For this review, take the finished solid that the model builds, in its own axes (mm). Give positions to 0.01 mm unless a question says otherwise; leave off trailing zeros. Loops run counter-clockwise (first coordinate to the right, second up) from the corner with the lowest first, then second, coordinate; pieces in that order, holes last. Notation, with made-up numbers: (78.25, -7.75) - (124.25, -7.75) arc R11 ccw to (124.25, 5.25) - close; hole circle Ø2 at (88, 51.5). An arc over 180 degrees is marked (long way). Answer in a Markdown table with one row per item.
Autodesk Inventor part; units mm, degrees
ref_plane "YZ Plane" through (0, 0, 0) normal (1, 0, 0) x (0, 1, 0)
ref_plane "XZ Plane" through (0, 0, 0) normal (0, 1, 0) x (-1, 0, 0)
ref_plane "XY Plane" through (0, 0, 0) normal (0, 0, 1) x (1, 0, 0)
sketch "Sketch1" plane through (0, 0, 0) normal (0, 0, 1) x (1, 0, 0)
  line L0 (0, 0) -> (0, 79.375)
  line L1 (0, 79.375) -> (-50.8, 79.375)
  line L2 (-50.8, 79.375) -> (-50.8, 25.4)
  line L3 (-50.8, 25.4) -> (-50.8, 0)
  line L4 (-50.8, 0) -> (0, 0)
  circle A0 centre (-25.4, 53.975) radius 6.35
  dimension "d0" = 79.375
  dimension "d1" = 50.8
  dimension "d2" = 25.4
  dimension "d3" = 50.8
  dimension "d4" = 25.4
  dimension "d5" = 25.4
  dimension "d6" = 12.7
extrude "Extrusion1" add sketch "Sketch1" against normal blind 3.175
properties part number "gearmotor mounting plate"
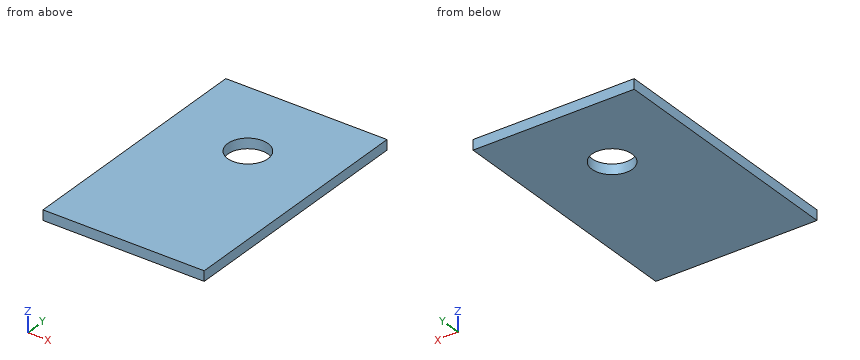
1. We need section C-C, the plane z = -2.6. Give the boundary of the cut face in (x, y) (3 decimals).
Values:
| item | result |
|---|---|
| outline | (-50.8, 0) - (0, 0) - (0, 79.375) - (-50.8, 79.375) - close; hole circle Ø12.7 at (-25.4, 53.975) |
2. Wall thickness on line 1 (Y direction, x = -25.4, z = -1.15) (3 decimals); line 2 (Y direction, x = -26, z = -2.45) (3 decimals); line 3 (X direction, y = 48.5, z = -1.3): over which ranges is each line inside the solid? List them lowest first. Write a range as [from, to].
Values:
| item | result |
|---|---|
| line 1 | y = [0, 47.625], [60.325, 79.375] |
| line 2 | y = [0, 47.653], [60.297, 79.375] |
| line 3 | x = [-50.8, -28.62], [-22.18, 0] |
3. We need section A-A, the plane x = -25.4. Give the boundary of the cut face in (y, z) (3 decimals), and give its area (3 significant figures).
Values:
| item | result |
|---|---|
| outline | (0, -3.175) - (47.625, -3.175) - (47.625, 0) - (0, 0) - close; (60.325, -3.175) - (79.375, -3.175) - (79.375, 0) - (60.325, 0) - close |
| area | 212 mm^2 |
4. We need section B-B, the plane y = 56. Give the boundary of the cut face in (x, z) (3 decimals), and give its area (3 significant figures).
Values:
| item | result |
|---|---|
| outline | (-50.8, -3.175) - (-31.418, -3.175) - (-31.418, 0) - (-50.8, 0) - close; (-19.382, -3.175) - (0, -3.175) - (0, 0) - (-19.382, 0) - close |
| area | 123 mm^2 |
